Source: CAD feature listing. Evaluate the final solid. Frame: model axes, mm. Face numbers are marked on the shaded views. A direction names the side the tool comes from. Give positions to 0.01 mm unless a question says otherwise; leave off trailing zeros. Order: outer loops, then holes, each group sorted by start corner. A loop starts at its lowest first (then second) coordinate and runs counter-clockwise, first axis right, second up. Notation, with made-up numbers: (34, 45) -> (72, 45) arc R21 ccw to (72, 71) -> close; hole circle Ø11 at (-2.75, -23). An arc over 180 degrees is marked (long way). Answer in a Markdown table with one row per item.
```python
from build123d import *

# Parameters (mm, degrees)
SZKIC1_W                    = 20
SZKIC1_H                    = 26
DODANIE_WYCI_GNI_CIE1_DEPTH = 5
SZKIC2_W                    = 20
SZKIC2_H                    = 6
DODANIE_WYCI_GNI_CIE2_DEPTH = 20
SZKIC3_W                    = 10.2
SZKIC3_H                    = 10.2
WYTNIJ_WYCI_GNI_CIE1_DEPTH  = 2
DODANIE_WYCI_GNI_CIE3_DEPTH = 20
SZKIC5_W                    = 10.2
SZKIC5_H                    = 10.2
WYTNIJ_WYCI_GNI_CIE2_DEPTH  = 5
SZKIC6_R                    = 2
WYTNIJ_WYCI_GNI_CIE3_DEPTH  = 6


with BuildPart() as part:
    # Szkic1 → Dodanie-wyciągnięcie1 (new body)
    with BuildSketch(Plane.XY):
        Rectangle(SZKIC1_W, SZKIC1_H)
    extrude(amount=DODANIE_WYCI_GNI_CIE1_DEPTH)

    # Szkic2 → Dodanie-wyciągnięcie2 (add)
    with BuildSketch(Plane(origin=(0, 0, 0), x_dir=(-1, 0, 0), z_dir=(0, 0, -1))):
        with Locations((0, 10)):
            Rectangle(SZKIC2_W, SZKIC2_H)
    extrude(amount=DODANIE_WYCI_GNI_CIE2_DEPTH)

    # Szkic3 → Wytnij-wyciągnięcie1 (cut)
    with BuildSketch(Plane.XY.offset(5)):
        with Locations((0, -6)):
            Rectangle(SZKIC3_W, SZKIC3_H)
    extrude(amount=-WYTNIJ_WYCI_GNI_CIE1_DEPTH, mode=Mode.SUBTRACT)

    # Szkic4 → Dodanie-wyciągnięcie3 (add)
    with BuildSketch(Plane(origin=(10, 0, 0), x_dir=(0, 0, -1), z_dir=(1, 0, 0))):
        Polygon((-5, 13), (20, 25.738136237), (20, 13), align=None)
    extrude(amount=-DODANIE_WYCI_GNI_CIE3_DEPTH)

    # Szkic5 → Wytnij-wyciągnięcie2 (cut)
    with BuildSketch(Plane(origin=(0, 12.343146626, 6.289147333), x_dir=(1, 0, 0), z_dir=(0, 0.8910065241883706, 0.4539904997395416))):
        with Locations((0, 16.446843876)):
            Rectangle(SZKIC5_W, SZKIC5_H)
    extrude(amount=-WYTNIJ_WYCI_GNI_CIE2_DEPTH, mode=Mode.SUBTRACT)

    # Szkic6 → Wytnij-wyciągnięcie3 (cut)
    with BuildSketch(Plane(origin=(0, 0, -20), x_dir=(-1, 0, 0), z_dir=(0, 0, -1))):
        with Locations((0, 13)):
            Circle(SZKIC6_R)
    extrude(amount=-WYTNIJ_WYCI_GNI_CIE3_DEPTH, mode=Mode.SUBTRACT)


solid = part.part
```
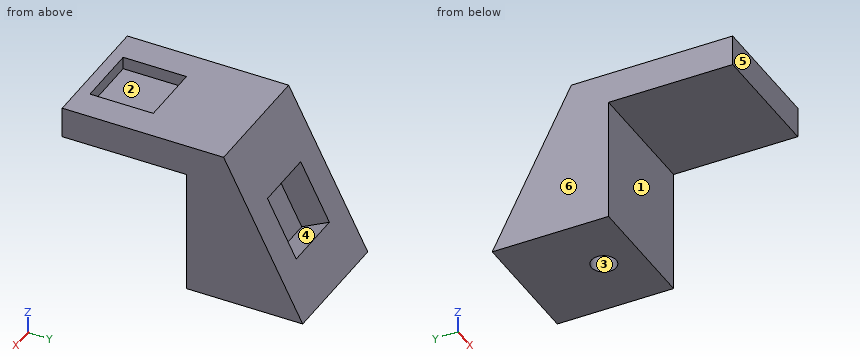
(1) Section query B-B (z = -13.5). Return the cut outline in (x, y).
A:
| item | result |
|---|---|
| outline | (-10, 7) -> (10, 7) -> (10, 22.43) -> (-10, 22.43) -> close; hole (-5.1, 16.81) -> (5.1, 16.81) -> (5.1, 20.97) -> (-5.1, 20.97) -> close |
(2) Ray query, probe 1 along Z at (x, y) = (5.75, -9.5); probe 2 along Y at (x, z) = (0, -17.25); probe 3 along Y at (x, z) = (3, 3.5). Return the intervals inside material, ascending.
A:
| item | result |
|---|---|
| probe 1 | z = 0 to 5 |
| probe 2 | y = 7 to 11, 15 to 24.34 |
| probe 3 | y = -13 to -11.1, -0.9 to 13.76 |
(3) First-contact query: pin 1 Ø5 at (y, z) = (-6, -1.5) entering from -X; pin 2 Ø2.5 at (x, y) = (0, 13) entering from -Z; pin 3 Ø1 at (x, z) = (-3, -7.5) entering from -Y; pin 4 Ø10 at (x, z) = (-1.5, 2) entering from +Y. Flat tips, straight axial feed; report the tip coordinate or a pass-through.
A:
| item | result |
|---|---|
| pin 1 | stops at x = -10 |
| pin 2 | stops at z = -14 |
| pin 3 | stops at y = 7 |
| pin 4 | stops at y = 17.08 |
(4) Section query D-D (y = 17). Return the cut outline in (x, z).
A:
| item | result |
|---|---|
| outline | (-10, -20) -> (10, -20) -> (10, -2.85) -> (-10, -2.85) -> close; hole (-5.1, -13.86) -> (5.1, -13.86) -> (5.1, -4.07) -> (-5.1, -4.07) -> close |
(5) Pull-direction query (Y, two-part tool) for the marked faces 4, 5 and 6; classes: +Y half, -Y half, draft (parallel to the pull), parting line (faces both ways), or undercut.
A:
| item | result |
|---|---|
| face 4 | undercut |
| face 5 | -Y half |
| face 6 | draft |
(6) Access query for the marked faces 1, 2 and 3. Directions: +Z, -Z, +X, -X, +Y, -Y. A direction counts if a zero-diameter tool reaches every point of the face in a straight line with its end or side. Return the directions, or none.
A:
| item | result |
|---|---|
| face 1 | -Z, +X, -X, -Y |
| face 2 | +Z |
| face 3 | -Z |
(7) Section query C-C (y = -8). Return the cut outline in (x, z).
A:
| item | result |
|---|---|
| outline | (-10, 0) -> (10, 0) -> (10, 5) -> (5.1, 5) -> (5.1, 3) -> (-5.1, 3) -> (-5.1, 5) -> (-10, 5) -> close |
(8) Section query A-A (x = 0). Return the cut outline in (y, z).
A:
| item | result |
|---|---|
| outline | (-13, 0) -> (7, 0) -> (7, -20) -> (11, -20) -> (11, -14) -> (15, -14) -> (15, -20) -> (25.74, -20) -> (22.13, -12.91) -> (17.67, -15.18) -> (13.04, -6.09) -> (17.49, -3.82) -> (13, 5) -> (-0.9, 5) -> (-0.9, 3) -> (-11.1, 3) -> (-11.1, 5) -> (-13, 5) -> close |
